Source: CAD feature listing. Evaluate the final solid. Frame: model axes, mm. Face numbers are marked on the shaded views. A direction names the side the tool comes from. Round coordinates to 2 decimals unless told otherwise and drop trailing zeros. Loops run counter-clockwise (first coordinate to the right, second up) from the corner with the lowest first, then second, coordinate; pieces in that order, holes last. Notation, with made-up numbers: (45, 75.25) - (103, 75.25) arc R24 ccw to (103, 102.25) - close; hole circle Ø3 at (67.5, -31). An arc over 180 degrees is marked (long way). One line per question, with ' | ' between items.
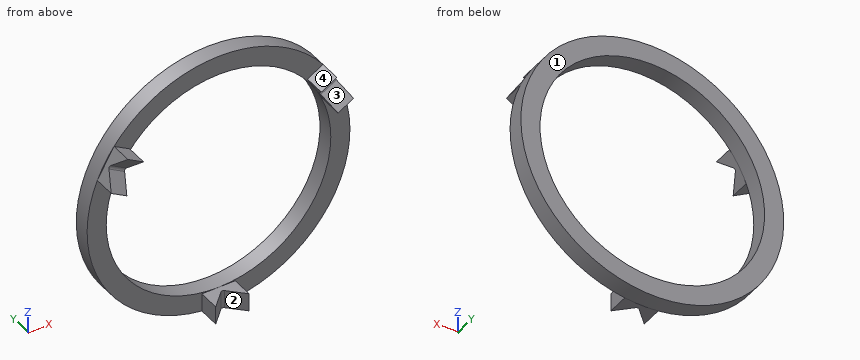
from build123d import *

# Parameters (mm, degrees)
SKETCH1_R                = 13.97
SKETCH1_R_2              = 11.938
BOSS_EXTRUDE1_DEPTH      = 1.778
BOSS_EXTRUDE2_DEPTH      = 2.286
CUT_EXTRUDE1_DEPTH       = 2.54
FILLET2_R                = 0.254
CIRPATTERN2_COUNT        = 3
FILLET2_OF_CIRPATTERN2_R = 0.254


with BuildPart() as part:
    # Sketch1 → Boss-Extrude1 (new body)
    with BuildSketch(Plane(origin=(0, 0, 0), x_dir=(1, 0, 0), z_dir=(0, 1, 0))):
        with Locations(Location((0, 0, 0), (0, 0, 270))):
            Circle(SKETCH1_R)
        with Locations(Location((0, 0, 0), (0, 0, 270))):
            Circle(SKETCH1_R_2, mode=Mode.SUBTRACT)
    extrude(amount=BOSS_EXTRUDE1_DEPTH)

    # Sketch3 → Boss-Extrude2 (add)
    with BuildSketch(Plane(origin=(0, 0, 0), x_dir=(-1, 0, 0), z_dir=(0, -1, 0))):
        Polygon((0, 11.938), (-1.778, 11.938), (-1.778, 13.856392604), (1.778, 13.856392604), (1.778, 11.938), align=None)
    boss_extrude2 = extrude(amount=BOSS_EXTRUDE2_DEPTH)

    # Sketch4 → Cut-Extrude1 (cut)
    with BuildSketch(Plane.XY.offset(-11.938)):
        Polygon((-1.778, -2.286), (0, -0.508), (1.778, -2.286), align=None)
    cut_extrude1 = extrude(amount=-CUT_EXTRUDE1_DEPTH, mode=Mode.SUBTRACT)

    # Fillet2
    fillet2_edges = [part.edges().sort_by_distance(p)[0] for p in [
        (0, -0.508, -12.897196302),
    ]]
    fillet(fillet2_edges, radius=FILLET2_R)

    # CirPattern2: Boss-Extrude2, Cut-Extrude1 ×3 about axis
    cirpattern2_axis = Axis((0, 0, 0), (0, 1, 0))
    add([boss_extrude2.rotate(cirpattern2_axis, i * 360 / CIRPATTERN2_COUNT) for i in range(1, CIRPATTERN2_COUNT)])
    add([cut_extrude1.rotate(cirpattern2_axis, i * 360 / CIRPATTERN2_COUNT) for i in range(1, CIRPATTERN2_COUNT)], mode=Mode.SUBTRACT)

    # Fillet2 of CirPattern2
    fillet2_of_cirpattern2_edges = [part.edges().sort_by_distance(p)[0] for p in [
        (-11.169299635, -0.508, 6.448598151),
        (11.169299635, -0.508, 6.448598151),
    ]]
    fillet(fillet2_of_cirpattern2_edges, radius=FILLET2_OF_CIRPATTERN2_R)


solid = part.part
1. Section query A-A, the plane z = 0. Return loops of the section in (x, y), plus the area to 3 significant figures.
Worked out:
outline: (-13.97, 0) - (-11.94, 0) - (-11.94, 1.78) - (-13.97, 1.78) - close; (11.94, 0) - (13.97, 0) - (13.97, 1.78) - (11.94, 1.78) - close | area: 7.23 mm2
2. Mould query, pull axis X, two halves, no side actions, for the marked faces 1 and 2. Classes: released by +X, released by -X, zero draft, split by the parting line, or undercut.
Worked out:
face 1: zero draft | face 2: undercut
3. Material intervals for probe 1 along X at (y, z) = (1.4, 0); probe 2 along Y at (x, z) = (-8.25, 9.5); probe 3 along Z at (x, y) = (-3.5, 0.6), sorted ascending.
Worked out:
probe 1: x = -13.97 to -11.94, 11.94 to 13.97 | probe 2: y = 0 to 1.78 | probe 3: z = -13.52 to -11.41, 11.41 to 13.52
4. Access query for the marked faces 3 and 4. Directions: +Z, -Z, +X, -X, +Y, -Y. A direction counts if a zero-diameter tool reaches every point of the face in a straight line with its end or side. Return the directions, or none.
Worked out:
face 3: -Y | face 4: +Z, -Y
5. Contact query for flat-ended pins moving along their axis: P1, Ø1.1, axis at x = -0.5, y = -1, coming from the -Z side; P2, Ø1, axis at y = 0, z = -6, coming from the +X side; P3, Ø2, axis at x = 12, z = 7, coming from the -Y side; P4, Ø4, axis at x = -7, z = -5, coming from the -Y side. Output: stop coordinate, or through.
Worked out:
P1: stops at z = -13.86 | P2: stops at x = 12.84 | P3: stops at y = -1.57 | P4: passes through
6. Section query D-D, the plane y = 0.9. Return loops of the section in (x, z).
Worked out:
outline: circle Ø27.94 at (0, 0); hole circle Ø23.88 at (0, 0)
7. Section query C-C, the plane y = -1.6. Return loops of the section in (x, z).
Worked out:
outline: (-12.89, 5.39) - (-11.23, 4.43) - (-10.88, 5.02) - (-12.55, 5.98) - close; (-11.45, 7.87) - (-9.79, 6.91) - (-9.45, 7.51) - (-11.11, 8.47) - close; (-1.78, -13.86) - (-1.09, -13.86) - (-1.09, -11.94) - (-1.78, -11.94) - close; (1.09, -13.86) - (1.78, -13.86) - (1.78, -11.94) - (1.09, -11.94) - close; (9.45, 7.51) - (9.79, 6.91) - (11.45, 7.87) - (11.11, 8.47) - close; (10.88, 5.02) - (11.23, 4.43) - (12.89, 5.39) - (12.55, 5.98) - close
